Build history of the part. All positions in model axes, mm. Round coordinates to 2 decimals unless told otherwise and drop trailing zeros. Order: outer loops, then holes, each group sorted by start corner. A loop starts at its lowest first (then second) coordinate and runs counter-clockwise, first axis right, second up. Notation, with made-up numbers: M 28,-35.5 L 34,-35.5 A29 cw 34,-12.5 Z; hole C 9,3 d8. An arc over 180 degrees is marked long. One line per item, written item: value. Start each with the question number.
Item 1: Band-saw the part on A-A, the plane z = 2740. Write the cut outline in (x, y).
Item 2: Band-saw the part on B-B, the plane x = 24.5. Write the cut outline in (y, z), then the cut area to 3 significant figures.
Item 3: Band-saw the part on C-C, the plane y = -8. Write the cut outline in (x, z).
Item 4: Probe L1, parallel to Y at x = 9, z = 2515; L2, parallel to Y at x = 14, z = 573; L3, parallel to X at y = 19, z = 2129.5. List the from-to ranges inside material, lowest first.
Autodesk Inventor part; units mm, degrees
ref_plane "Начальная плоскость" through (0, 0, 40) normal (0, 0, 1) x (1, 0, 0)
ref_plane "Конечная плоскость" through (0, 0, 3030) normal (0, 0, 1) x (1, 0, 0)
ref_plane "РабПлоскость4" through (-1.43, 1220, 40) normal (0, 0, -1) x (-1, 0, 0)
ref_plane "Начальная плоскость" through (0, 0, 40) normal (0, 0, 1) x (1, 0, 0)
ref_plane "Конечная плоскость" through (0, 0, 3030) normal (0, 0, 1) x (1, 0, 0)
sketch "Эскиз" plane through (0, 0, 0) normal (0, 0, 1) x (1, 0, 0)
  line L0 (-1.43, 0) -> (-1.43, 40)
  line L1 (-1.43, 40) -> (43.57, 40)
  line L2 (43.57, 40) -> (43.57, 38.1774)
  line L3 (39.9881, 34.1993) -> (11.2338, 31.1771)
  line L4 (4.07, 23.221) -> (4.07, 0)
  line L5 (4.07, 0) -> (-1.43, 0) construction
  line L6 (23.82, 40) -> (23.82, 32.5) construction
  line L7 (43.57, 34.5758) -> (43.57, 32.5) construction
  line L8 (43.57, 32.5) -> (23.82, 32.5) construction
  line L9 (0, 15) -> (0, -27) construction
  line L10 (-5.539, 0) -> (16.0067, 0) construction
  line L11 (-1.43, 0) -> (-1.43, -40)
  line L12 (-1.43, -40) -> (43.57, -40)
  line L13 (43.57, -40) -> (43.57, -38.1774)
  line L14 (39.9881, -34.1993) -> (11.2338, -31.1771)
  line L15 (4.07, -23.221) -> (4.07, 0)
  arc A0 (11.2338, 31.1771) -> (4.07, 23.221) centre (12.07, 23.221) ccw
  arc A1 (4.07, -23.221) -> (11.2338, -31.1771) centre (12.07, -23.221) ccw
  arc A2 (39.9881, 34.1993) -> (43.57, 38.1774) centre (39.57, 38.1774) ccw
  arc A3 (43.57, -38.1774) -> (39.9881, -34.1993) centre (39.57, -38.1774) ccw
  line L16 (0, 56) -> (0, -56) construction
  line L17 (-15.5135, 0) -> (54.308, 0) construction
  point P0 (4.07, 30.4242)
  point P1 (43.57, -34.5758)
  point P2 (4.07, -30.4242)
  point P3 (23.82, -40)
  point P4 (23.82, -32.5)
  dimension "d0" = 5.5
  dimension "d1" = 40
  dimension "d2" = 45
  dimension "d3" = 7.5
  dimension "d4" = 19.75
  dimension "d5" = 2.0758
  dimension "d23" = 8
  dimension "d24" = 4
  dimension "d25" = 1.43
extrude "Тело" add sketch "Эскиз" along normal up to surface (2990 mm away) from surface at 40
sketch "Sketch3" plane through (0, 0, 0) normal (0, 0, 1) x (1, 0, 0)
  line L0 (0, 0) -> (10, 0)
ref_plane "Work Plane3" through (0, 0, 0) normal (0, -1, 0) x (1, 0, 0)
sketch "Sketch4" plane through (0, 0, 0) normal (0, -1, 0) x (1, 0, 0)
  line L0 (-2, 40) -> (12, 40)
  line L1 (-2, 3030) -> (12, 3030)
  dimension "d29" = 2990
ref_plane "РабПлоскость4" through (-1.43, 1220, 40) normal (0, 0, -1) x (-1, 0, 0)
split "Разделение1" plane through (-1.43, 1220, 40) removes the side toward (0, 0, -1)
ref_plane "РабПлоскость5" through (-1.43, -500, 3030) normal (0, 0, 1) x (1, 0, 0)
split "Разделение2" plane through (-1.43, -500, 3030) removes the side toward (0, 0, 1)
equation "\"d0\" = G_T"
equation "\"d1\" = 0.5 * G_H"
equation "\"d2\" = G_W"
equation "\"d3\" = G_T1"
equation "\"d4\" = G_C"
equation "\"d23\" = G_IR"
equation "\"d24\" = G_ER"
equation "\"d25\" = ex"
equation "\"d6\" = G_L"
equation "\"G_W\" = 45"
equation "\"G_T\" = 5.5"
equation "\"G_T1\" = 7.5"
equation "\"G_NG\" = 0.105104"
equation "\"G_ER\" = 4"
equation "\"G_IR\" = 8"
equation "\"G_C\" = 19.75"
equation "\"G_L\" = d29"
equation "\"ex\" = 1.43"
properties part number "ISO 657/11 - CH 80 x 8 - 2990" material "Сталь, мягкая"
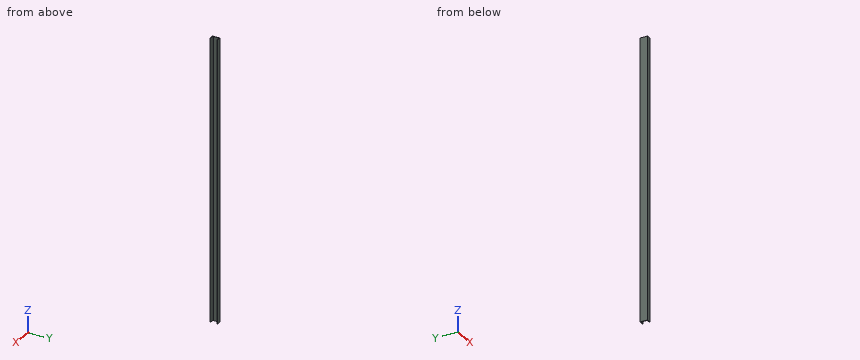
Output:
1. outline: M -1.43,-40 L 43.57,-40 L 43.57,-38.18 A4 ccw 39.99,-34.2 L 11.23,-31.18 A8 cw 4.07,-23.22 L 4.07,23.22 A8 cw 11.23,31.18 L 39.99,34.2 A4 ccw 43.57,38.18 L 43.57,40 L -1.43,40 Z
2. outline: M -40,40 L -32.57,40 L -32.57,3030 L -40,3030 Z; M 32.57,40 L 40,40 L 40,3030 L 32.57,3030 Z
2. area: 44,400 mm²
3. outline: M -1.43,40 L 4.07,40 L 4.07,3030 L -1.43,3030 Z
4. L1: y = -40 to -30.61, 30.61 to 40
4. L2: y = -40 to -31.47, 31.47 to 40
4. L3: x = -1.43 to 4.07
